```python
from build123d import *

# Parameters (mm, degrees)
F0_W     = 187
F0_H     = 38.963933
F0_R     = 1.7
F0_W_2   = 33.4
F0_H_2   = 16.5
F0_R_2   = 7.5
F1_DEPTH = 2.35


with BuildPart() as f1:
    # F0 (on Top) → F1 (new body)
    with BuildSketch(Plane.XY):
        with Locations((10.5, -0.518033)):
            Rectangle(F0_W, F0_H)
        with Locations((-22.675, -6.4)):
            Circle(F0_R, mode=Mode.SUBTRACT)
        with Locations((-3.3, -2.65)):
            Rectangle(F0_W_2, F0_H_2, mode=Mode.SUBTRACT)
        with Locations((16.075, -6.4)):
            Circle(F0_R, mode=Mode.SUBTRACT)
        with Locations((-70, 0)):
            Circle(F0_R_2, mode=Mode.SUBTRACT)
        with Locations((-22.675, 1.1)):
            Circle(F0_R, mode=Mode.SUBTRACT)
        with Locations((16.075, 1.1)):
            Circle(F0_R, mode=Mode.SUBTRACT)
        with Locations((70, 0)):
            Circle(F0_R_2, mode=Mode.SUBTRACT)
    extrude(amount=F1_DEPTH)


solid = f1.part
```
Could you check a few things on this model? Use its own coordinates, in mm. Round coordinates to 2 decimals unless told otherwise and drop trailing zeros. Loops run counter-clockwise (first coordinate to the right, second up) from the corner with the lowest first, then second, coordinate; pieces in that order, holes last. Notation, with made-up numbers: (-15.75, 49) -> (2.25, 49) arc R26 cw to (2.25, 72) -> close; hole circle Ø7 at (83.25, 37.25). An arc over 180 degrees is marked (long way). One line per question, with ' | ' between items.
(1) Thinking about a two-plate mould opening in Y: for faces 1 (the face through (-77.493, 0.33, 1.159)), 2 (the face through (9, 8, 2.35)), 3 (the face through (-21.054, -5.889, 1.159)), which applies, released by +Y, released by -Y, zero draft, split by the parting line, or undercut?
Model answer:
face 1: undercut | face 2: zero draft | face 3: undercut
(2) If we section it at C-C on y = -2.5: List the corners of the cut face in (x, z) for me.
Model answer:
outline: (-83, 0) -> (-77.07, 0) -> (-77.07, 2.35) -> (-83, 2.35) -> close; (-62.93, 0) -> (-20, 0) -> (-20, 2.35) -> (-62.93, 2.35) -> close; (13.4, 0) -> (62.93, 0) -> (62.93, 2.35) -> (13.4, 2.35) -> close; (77.07, 0) -> (104, 0) -> (104, 2.35) -> (77.07, 2.35) -> close
(3) If we section it at A-A on z = 1: List the corners of the cut face in (x, y) for me (3 decimals), and give its area (3 significant figures).
Model answer:
outline: (-83, -20) -> (104, -20) -> (104, 18.964) -> (-83, 18.964) -> close; hole circle Ø15 at (-70, 0); hole circle Ø3.4 at (-22.675, -6.4); hole circle Ø3.4 at (-22.675, 1.1); hole (-20, -10.9) -> (13.4, -10.9) -> (13.4, 5.6) -> (-20, 5.6) -> close; hole circle Ø3.4 at (16.075, -6.4); hole circle Ø3.4 at (16.075, 1.1); hole circle Ø15 at (70, 0) | area: 6,350 mm^2
(4) If I drill on probe 1 along Y at (x, z) = (-9, 1.1); probe 2 along Y at (x, z) = (70, 1.6); probe 3 along X at (y, z) = (-10, 0.3), over which ranges is the centre line in solid material (lowest first)?
Model answer:
probe 1: y = -20 to -10.9, 5.6 to 18.96 | probe 2: y = -20 to -7.5, 7.5 to 18.96 | probe 3: x = -83 to -20, 13.4 to 104
(5) If we section it at D-D on x = 70: List the corners of the cut face in (y, z) for me, and give its area (3 significant figures).
Model answer:
outline: (-20, 0) -> (-7.5, 0) -> (-7.5, 2.35) -> (-20, 2.35) -> close; (7.5, 0) -> (18.96, 0) -> (18.96, 2.35) -> (7.5, 2.35) -> close | area: 56.3 mm^2
(6) If we section it at B-B on x = -16.5: List the corners of the cut face in (y, z) for me, and give its area (3 significant figures).
Model answer:
outline: (-20, 0) -> (-10.9, 0) -> (-10.9, 2.35) -> (-20, 2.35) -> close; (5.6, 0) -> (18.96, 0) -> (18.96, 2.35) -> (5.6, 2.35) -> close | area: 52.8 mm^2
